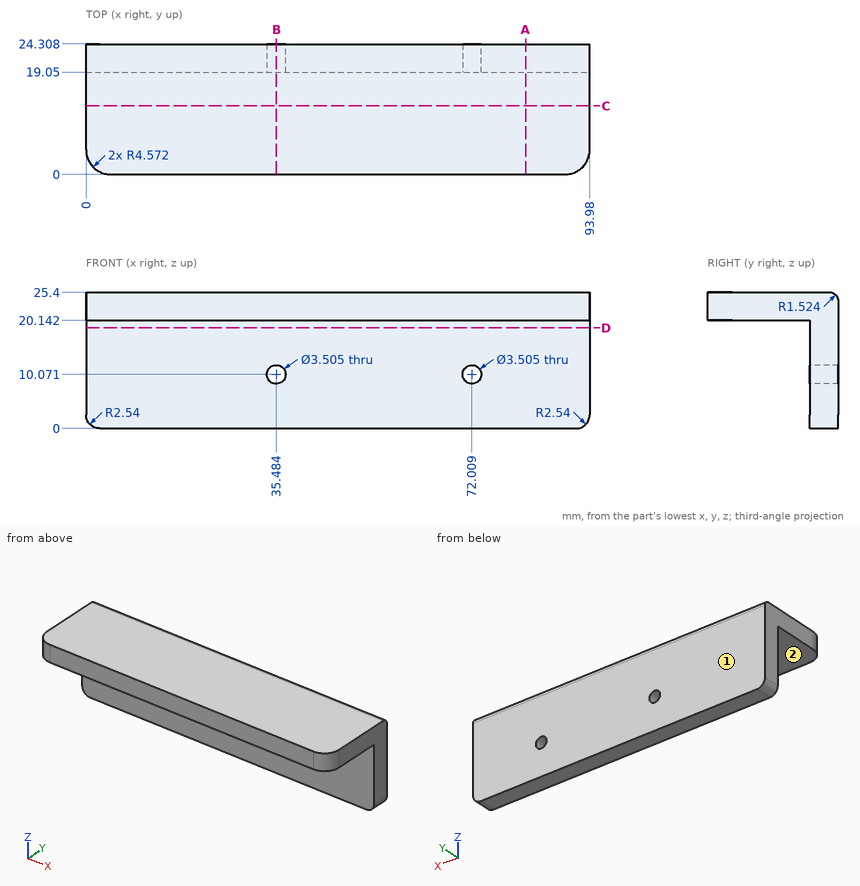
Study the drawing (mm; zero at the part's minimum x, y, z) and answer. A direction names the side the tool comes from. Give positions to 0.01 mm unless a question says otherwise; leave off trailing zeros. Write each loop counter-clockwise with the first axis right and the second up, starting at its lowest first coordinate (ties: lowest second). Pieces come first, ordered by that corner, then holes.
Item 1: Section D-D, the plane z = 18.75 is taken. Write down the section's boundary in (x, y), plus the area to 3 significant figures.
Item 2: Section A-A, the plane x = 82 is taken. Write down the section's boundary in (y, z), plus the area to 3 significant figures.
Item 3: Which of the six approach directions +Z, -Z, +X, -X, +Y, -Y give full straight-line access (tool end or side, diameter ignored) to the marked faces 1 and 2?
Item 4: Section B-B, the plane x = 35.5 is taken. Write down the section's boundary in (y, z).
Item 5: Section C-C, the plane y = 12.75 is taken. Write down the section's boundary in (x, z).
Item 6: Find the intervals of material crossed by line 1 along X through (y, z) = (22, 10) (1 decimal); line 2 along Y through (x, z) = (55, 2.25); line 3 along Z through (x, y) = (61.5, 15.75), in increasing order.
Item 7: Flat-ended cylindrical pins translate along their axes: P1, Ø4.5, axis at x = 72.01, z = 10.07, coming from the +Y side; P2, Ø2, axis at x = 22, y = 14, coming from the -Z side; P3, Ø5.5, axis at x = 35.48, z = 10.07, coming from the -Y side. Find the tip coordinate at first contact, or state that the pin passes through.
Completed:
1. outline: (0, 19.05) - (93.98, 19.05) - (93.98, 24.31) - (0, 24.31) - close
1. area: 494 mm2
2. outline: (0, 20.14) - (19.05, 20.14) - (19.05, 0) - (24.31, 0) - (24.31, 23.88) arc R1.52 ccw to (22.78, 25.4) - (0, 25.4) - close
2. area: 233 mm2
3. face 1: +Z, -Z, +X, -X, +Y
3. face 2: -Z, +X, -X, -Y
4. outline: (0, 20.14) - (19.05, 20.14) - (19.05, 11.82) - (24.31, 11.82) - (24.31, 23.88) arc R1.52 ccw to (22.78, 25.4) - (0, 25.4) - close; (19.05, 0) - (24.31, 0) - (24.31, 8.32) - (19.05, 8.32) - close
5. outline: (0, 20.14) - (93.98, 20.14) - (93.98, 25.4) - (0, 25.4) - close
6. line 1: x = 0 to 33.7, 37.2 to 70.3, 73.8 to 94
6. line 2: y = 19.05 to 24.31
6. line 3: z = 20.14 to 25.4
7. P1: stops at y = 24.31
7. P2: stops at z = 20.14
7. P3: stops at y = 19.05
